Geometry check sheet. Reference: the model listing, model coordinates, mm. Coordinates: 2 decimals unless noted, no trailing zeros. Write each loop counter-clockwise with the first axis right and the second up, starting at its lowest first coordinate (ties: lowest second). Pieces come first, ordered by that corner, then holes. Notation, with made-up numbers: (60, 5) -> (95, 5) arc R13 cw to (95, 30) -> close; hole circle Ø9 at (40, 81.5). An arc over 180 degrees is marked (long way). Answer as CSV lines item,"result".
```python
from build123d import *

# Parameters (mm, degrees)
CROQUIS1_W              = 55
CROQUIS1_H              = 55
CROQUIS1_R              = 3
CROQUIS1_R_2            = 1.25
SALIENTE_EXTRUIR1_DEPTH = 2
REDONDEO1_R             = 5
CORTAR_EXTRUIR1_DEPTH   = 2


with BuildPart() as part:
    # Croquis1 → Saliente-Extruir1 (new body)
    with BuildSketch(Plane.XY):
        Rectangle(CROQUIS1_W, CROQUIS1_H)
        with Locations((-22.550252532, 22.550252532)):
            Circle(CROQUIS1_R, mode=Mode.SUBTRACT)
        with Locations((22.550252532, 22.550252532)):
            Circle(CROQUIS1_R, mode=Mode.SUBTRACT)
        with Locations((22.550252532, -22.550252532)):
            Circle(CROQUIS1_R, mode=Mode.SUBTRACT)
        with Locations((-22.550252532, -22.550252532)):
            Circle(CROQUIS1_R, mode=Mode.SUBTRACT)
        Circle(CROQUIS1_R, mode=Mode.SUBTRACT)
        with Locations((-6.717514421, 6.717514421)):
            Circle(CROQUIS1_R_2, mode=Mode.SUBTRACT)
        with Locations((6.717514421, 6.717514421)):
            Circle(CROQUIS1_R_2, mode=Mode.SUBTRACT)
        with Locations((6.717514421, -6.717514421)):
            Circle(CROQUIS1_R_2, mode=Mode.SUBTRACT)
        with Locations((-6.717514421, -6.717514421)):
            Circle(CROQUIS1_R_2, mode=Mode.SUBTRACT)
    extrude(amount=SALIENTE_EXTRUIR1_DEPTH)

    # Redondeo1
    redondeo1_edges = [part.edges().sort_by_distance(p)[0] for p in [
        (27.5, -27.5, 1),
        (-27.5, -27.5, 1),
        (-27.5, 27.5, 1),
        (27.5, 27.5, 1),
    ]]
    fillet(redondeo1_edges, radius=REDONDEO1_R)

    # Croquis2 → Cortar-Extruir1 (cut)
    with BuildSketch(Plane.XY.offset(2)):
        with BuildLine():
            ThreePointArc((-26.035533906, -26.035533906), (-27.103992097, -20.664031844), (-22.550252532, -17.621320344))
            ThreePointArc((-22.550252532, -17.621320344), (-14.66565297, 0), (-22.550252532, 17.621320344))
            ThreePointArc((-22.550252532, 17.621320344), (-27.103991999, 20.664031606), (-26.03553427, 26.035533542))
            ThreePointArc((-26.03553427, 26.035533542), (-27.119397761, 24.413416924), (-27.5, 22.5))
            Line((-27.5, 22.5), (-27.5, -22.5))
            ThreePointArc((-27.5, -22.5), (-27.119397663, -24.413417162), (-26.035533906, -26.035533906))
        make_face()
        with BuildLine():
            ThreePointArc((-22.5, 27.5), (-24.4134174, 27.119397564), (-26.03553427, 26.035533542))
            ThreePointArc((-26.03553427, 26.035533542), (-20.664032082, 27.103992196), (-17.621320344, 22.550252532))
            ThreePointArc((-17.621320344, 22.550252532), (0, 14.66565297), (17.621320344, 22.550252532))
            ThreePointArc((17.621320344, 22.550252532), (20.664031651, 27.103992018), (26.035533611, 26.035534201))
            ThreePointArc((26.035533611, 26.035534201), (24.413416969, 27.119397742), (22.5, 27.5))
            Line((22.5, 27.5), (-22.5, 27.5))
        make_face()
        with BuildLine():
            ThreePointArc((22.550252532, -17.621320344), (27.10399228, -20.664032285), (26.03553323, -26.035534581))
            ThreePointArc((26.03553323, -26.035534581), (27.11939748, -24.413417603), (27.5, -22.5))
            Line((27.5, -22.5), (27.5, 22.5))
            ThreePointArc((27.5, 22.5), (27.119397583, 24.413417354), (26.035533611, 26.035534201))
            ThreePointArc((26.035533611, 26.035534201), (27.103992177, 20.664032037), (22.550252532, 17.621320344))
            ThreePointArc((22.550252532, 17.621320344), (14.66565297, 0), (22.550252532, -17.621320344))
        make_face()
        with BuildLine():
            ThreePointArc((-17.621320344, -22.550252532), (-20.664031844, -27.103992097), (-26.035533906, -26.035533906))
            ThreePointArc((-26.035533906, -26.035533906), (-24.413417162, -27.119397663), (-22.5, -27.5))
            Line((-22.5, -27.5), (22.5, -27.5))
            ThreePointArc((22.5, -27.5), (24.413416721, -27.119397845), (26.03553323, -26.035534581))
            ThreePointArc((26.03553323, -26.035534581), (20.664031403, -27.103991915), (17.621320344, -22.550252532))
            ThreePointArc((17.621320344, -22.550252532), (0, -14.66565297), (-17.621320344, -22.550252532))
        make_face()
    extrude(amount=-CORTAR_EXTRUIR1_DEPTH, mode=Mode.SUBTRACT)


solid = part.part
```
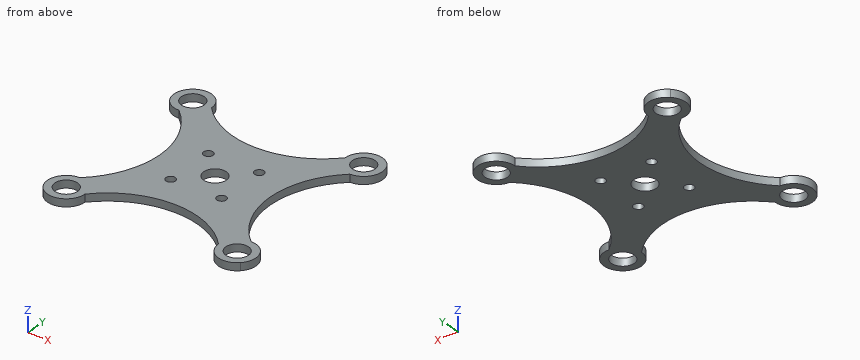
Item 1: Cross-section at C-C, the plane y = -21. Record the cut outline in (x, z), plus the area to 3 significant figures.
Responses:
outline,"(-27.23, 0) -> (-25.12, 0) -> (-25.12, 2) -> (-27.23, 2) -> close; (-19.98, 0) -> (-16.1, 0) -> (-16.1, 2) -> (-19.98, 2) -> close; (16.1, 0) -> (19.98, 0) -> (19.98, 2) -> (16.1, 2) -> close; (25.12, 0) -> (27.23, 0) -> (27.23, 2) -> (25.12, 2) -> close"
area,"24.0 mm2"
Item 2: Cross-section at D-D, the plane z = 1.3. Count the separate pieces of the cut face and the enclosed holes in it, plus the area to 3 significant figures.
Responses:
separate pieces,"1"
enclosed holes,"9"
area,"1,330 mm2"
Item 3: Cross-section at A-A, the plane y = 0. Record the cut outline in (x, z), plus the area to 3 significant figures.
Responses:
outline,"(-14.67, 0) -> (-3, 0) -> (-3, 2) -> (-14.67, 2) -> close; (3, 0) -> (14.67, 0) -> (14.67, 2) -> (3, 2) -> close"
area,"46.7 mm2"
Item 4: Thickness scan on probe 1 along Y at (x, z) = (-23, 0.5); probe 2 along Y at (x, z) = (-20.5, 1.75); probe 3 along Y at (x, z) = (-7, 1.05). Record the ranges inside material, lowest first.
Responses:
probe 1,"y = -27.46 to -25.52, -19.58 to -17.64, 17.64 to 19.58, 25.52 to 27.46"
probe 2,"y = -27.03 to -24.74, -20.36 to -15.55, 15.55 to 20.36, 24.74 to 27.03"
probe 3,"y = -15.73 to -7.94, -5.5 to 5.5, 7.94 to 15.73"
Item 5: Depth check by flat-ended pin: pin 1 Ø8 at (x, y) = (-22.55, 22.55) entering from +Z; pin 2 Ø3.5 at (x, y) = (0, 0) entering from -Z; pin 3 Ø1 at (x, z) = (20.5, 0.5) entering from -Y. Enter the tip coordinate at first touch or a pass-through.
Responses:
pin 1,"stops at z = 2"
pin 2,"passes through"
pin 3,"stops at y = -27.23"
